Could you check a few things on this model? Use its own coordinates, in mm. A direction names the side the tool comes from. Round coordinates to 2 decimals unless told otherwise and drop trailing zeros. Write each loop counter-clockwise with the first axis right and the second up, starting at its lowest first coordinate (ties: lowest second). Pieces come first, ordered by that corner, then holes. Notation, with made-up numbers: (-30.5, 61) -> (-22.5, 61) arc R18 cw to (-22.5, 77) -> close; hole circle Ø7 at (-32, 24). An arc over 180 degrees is marked (long way). Return JSON: item names as keys, results as strings.
Autodesk Inventor part; units mm, degrees
ref_plane "YZ Plane" through (0, 0, 0) normal (1, 0, 0) x (0, 1, 0)
ref_plane "XZ Plane" through (0, 0, 0) normal (0, 1, 0) x (-1, 0, 0)
ref_plane "XY Plane" through (0, 0, 0) normal (0, 0, 1) x (1, 0, 0)
sketch "Sketch1" plane through (0, 0, 0) normal (0, 0, 1) x (1, 0, 0)
  arc A0 (37.7266, -9.8844) -> (-37.7266, -9.8844) centre (0, 0) ccw
  arc A1 (-34.0962, -52.1712) -> (-21.585, -59.437) centre (-26.125, -52.85) ccw
  arc A2 (21.585, -59.437) -> (34.0962, -52.1712) centre (26.125, -52.85) ccw
  arc A3 (-34.0962, -52.1712) -> (-37.7266, -9.8844) centre (-158.6454, -41.565) ccw
  line L0 (0, 64.9508) -> (0, -116.7047)
  arc A4 (21.585, -59.437) -> (-21.585, -59.437) centre (0, -90.7539) ccw
  arc A5 (37.7266, -9.8844) -> (34.0962, -52.1712) centre (158.6454, -41.565) ccw
  dimension "d0" = 16
  dimension "d2" = 78
  dimension "d3" = 52.85
  dimension "d5" = 26.125
  dimension "d8" = 317.2907
  dimension "d9" = 26.125
  dimension "d10" = 38.035
extrude "Extrusion1" add sketch "Sketch1" against normal blind 4
sketch "Sketch2" plane through (0, 0, -4) normal (0, 0, -1) x (-1, 0, 0)
  arc A0 (37.7266, -9.8844) -> (-37.7266, -9.8844) centre (0, 0) ccw
  arc A1 (-34.0962, -52.1712) -> (-21.585, -59.437) centre (-26.125, -52.85) ccw
  arc A2 (21.585, -59.437) -> (-21.585, -59.437) centre (0, -90.7539) ccw
  line L0 (-27.275, -50.4758) -> (-27.275, -48.2242)
  line L1 (-21.575, -51.5151) -> (-23.525, -52.6409)
  line L2 (-23.525, -46.0591) -> (-21.575, -47.1849)
  arc A3 (-23.525, -46.0591) -> (-27.275, -48.2242) centre (-24.775, -48.2242) ccw
  arc A4 (-27.275, -50.4758) -> (-23.525, -52.6409) centre (-24.775, -50.4758) ccw
  arc A5 (-21.575, -51.5151) -> (-21.575, -47.1849) centre (-22.825, -49.35) ccw
  line L3 (0, -116.7047) -> (0, 64.9508)
  point P0 (-27.275, 27.8761)
  point P1 (-32.4256, -57.7797)
  point P2 (-9.7764, -53.9968)
  dimension "d13" = 60
  dimension "d14" = 60
  dimension "d15" = 2.5
  dimension "d16" = 22.825
  dimension "d17" = 49.35
  dimension "d18" = 60
  dimension "d19" = 1.95
extrude "Extrusion2" add sketch "Sketch2" along normal blind 2.5
chamfer "Chamfer1" distance 2.5 angle 45 6 edges at (22.55, -52.078, -4) (26.025, -52.6409, -4) (27.275, -49.35, -4) (26.025, -46.0591, -4) (22.55, -46.622, -4) (20.325, -49.35, -4)
mirror "Mirror1" about plane through (0, 0, 0) normal (1, 0, 0) of "Extrusion2", "Chamfer1"
sketch "Sketch3" plane through (0, 0, 0) normal (0, 0, 1) x (1, 0, 0)
  line L0 (-23.525, -46.0591) -> (-21.575, -47.1849)
  arc A0 (-21.575, -51.5151) -> (-21.575, -47.1849) centre (-22.825, -49.35) ccw
  line L1 (-21.575, -51.5151) -> (-23.525, -52.6409)
  arc A1 (-27.275, -50.4758) -> (-23.525, -52.6409) centre (-24.775, -50.4758) ccw
  line L2 (-27.275, -50.4758) -> (-27.275, -48.2242)
  arc A2 (-23.525, -46.0591) -> (-27.275, -48.2242) centre (-24.775, -48.2242) ccw
  line L3 (-22.65, -54.1564) -> (-20.7, -53.0306)
  arc A3 (-20.7, -53.0306) -> (-20.7, -45.6694) centre (-22.825, -49.35) ccw
  line L4 (-20.7, -45.6694) -> (-22.65, -44.5436)
  arc A4 (-22.65, -44.5436) -> (-29.025, -48.2242) centre (-24.775, -48.2242) ccw
  line L5 (-29.025, -48.2242) -> (-29.025, -50.4758)
  arc A5 (-29.025, -50.4758) -> (-22.65, -54.1564) centre (-24.775, -50.4758) ccw
  dimension "d30" = 1.75
extrude "Extrusion3" cut sketch "Sketch3" against normal blind 2.5 contours L0 A0 L1 A1 L2 A2 | A5 L5 A4 L4 A3 L3
chamfer "Chamfer2" distance 2.5 angle 45 6 edges at (-26.9, -54.1564, -2.5) (-21.675, -53.5935, -2.5) (-18.575, -49.35, -2.5) (-21.675, -45.1065, -2.5) (-26.9, -44.5436, -2.5) (-29.025, -49.35, -2.5)
mirror "Mirror2" about plane through (0, 0, 0) normal (1, 0, 0) of "Extrusion3", "Chamfer2"
sketch "Sketch4" plane through (0, 0, 0) normal (0, 0, 1) x (1, 0, 0)
  circle A0 centre (0, 0) radius 8.5
  line L0 (0, 0) -> (0, -45)
  circle A1 centre (0, -45) radius 4
  dimension "d31" = 17
  dimension "d32" = 45
  dimension "d33" = 8
extrude "Extrusion4" cut sketch "Sketch4" against normal through all
sketch "Sketch5" plane through (0, 0, 0) normal (0, 0, 1) x (1, 0, 0)
  circle A0 centre (0, 0) radius 8.5
  line L0 (-29.025, -50.4758) -> (-29.025, -48.2242)
  arc A1 (37.7266, -9.8844) -> (-37.7266, -9.8844) centre (0, 0) ccw
  arc A2 (-2.8, 33.8845) -> (-33.908, 2.5) centre (0, 0) ccw
  arc A3 (-2.8, 19.803) -> (-19.8431, 2.5) centre (0, 0) ccw
  line L1 (-2.8, 33.8845) -> (-2.8, 19.803)
  line L2 (-19.8431, 2.5) -> (-33.908, 2.5)
  dimension "d36" = 68
  dimension "d37" = 40
  dimension "d38" = 2.5
  dimension "d39" = 2.8
extrude "Extrusion5" cut sketch "Sketch5" against normal blind 1.5 contours L1 A3 L2 A2
fillet "Fillet1" radius 6.75 4 edges at (-2.8, 33.8845, -0.75) (-2.8, 19.803, -0.75) (-19.8431, 2.5, -0.75) (-33.908, 2.5, -0.75)
pattern_circular "Circular Pattern1" count 4 over 360 about axis through (0, 0, 0) along (0, 0, -1) of "Extrusion5", "Fillet1"
properties part number "201-09" material "Steel"
1) Will these pins go through, and if not, where does the flat tip stop? pin 1 Ø2 at (x, z) = (16, -2) entering from +Y; pin 2 Ø7 at (x, y) = (0, -45) entering from -Z; pin 3 Ø2.5 at (x, y) = (22.5, -50) entering from +Z; pin 4 Ø0.6 at (x, z) = (25.5, -0.5) entering from -Y.
Return value:
{"pin 1": "y = 36", "pin 2": "through", "pin 3": "z = -2.28", "pin 4": "y = -60.84"}
2) If I drill on probe 1 along Y at (x, z) = (0, -2.5); probe 2 along X at (y, z) = (0, -0.8); probe 3 along Y at (x, z) = (-13.5, -1), over which ranges is the centre line in solid material (lowest first)? Write a range as [from, to].
Return value:
{"probe 1": "[-52.72, -49], [-41, -8.5], [8.5, 39]", "probe 2": "[-39, -8.5], [8.5, 39]", "probe 3": "[-55.2, -31.2], [-14.76, 14.76], [31.2, 36.59]"}
3) I want a section at A-A, the plane y = 0. Please give me the cut outline in (x, z).
Return value:
{"outline": "(-39, -4) -> (-8.5, -4) -> (-8.5, 0) -> (-39, 0) -> close; (8.5, -4) -> (39, -4) -> (39, 0) -> (8.5, 0) -> close"}
4) For faces 4 (the face through (24.046, 24.037, -0.74)), 5 (the face through (-34.08, -31.17, -1.97)), which set-ups out of +Z, -Z, +X, -X, +Y, -Y let a thin tool reach every point of the face, with its end or its side?
Return value:
{"face 4": "+Z", "face 5": "+Z, -Z, -X"}
5) I want a section at B-B, the plane x = 0. Please give me the cut outline in (y, z).
Return value:
{"outline": "(-52.72, -4) -> (-49, -4) -> (-49, 0) -> (-52.72, 0) -> close; (-41, -4) -> (-8.5, -4) -> (-8.5, 0) -> (-41, 0) -> close; (8.5, -4) -> (39, -4) -> (39, 0) -> (8.5, 0) -> close"}
6) Thinking about a two-plate mould opening in Y: for faces 1 (the face through (-20.085, -49.39, -1.51)), 2 (the face through (21.95, -53.15, -5.27)), 3 (the face through (-24, -49, -6.5)), which applies, pulls with the +Y half, pulls with the -Y half, needs draft (parallel to the pull), parting line crosses it, or undercut?
Return value:
{"face 1": "undercut", "face 2": "pulls with the -Y half", "face 3": "needs draft"}
